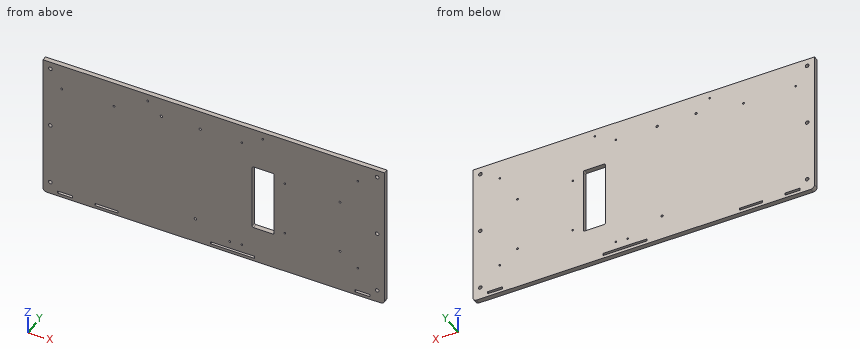
from build123d import *

# Parameters (mm, degrees)
SKETCH1_W           = 463.88
SKETCH1_H           = 192
BOSS_EXTRUDE1_DEPTH = 6.35
SKETCH5_R           = 2.5
CUT_EXTRUDE3_DEPTH  = 484.483469107
SKETCH4_R           = 1.25
SKETCH4_R_2         = 1.6
CUT_EXTRUDE2_DEPTH  = 484.483469107
SKETCH2_W           = 463.88
SKETCH2_H           = 7.175
BOSS_EXTRUDE2_DEPTH = 6.35
SKETCH3_W           = 20
SKETCH3_H           = 3.175
SKETCH3_W_2         = 31.25
SKETCH3_W_3         = 59.87
CUT_EXTRUDE1_DEPTH  = 484.483469107
FILLET1_R           = 5
SKETCH6_W           = 30
SKETCH6_H           = 92
CUT_EXTRUDE4_DEPTH  = 484.483469107
FILLET2_R           = 2


with BuildPart() as part:
    # Sketch1 → Boss-Extrude1 (new body)
    with BuildSketch(Plane(origin=(0, 0, 0), x_dir=(1, 0, 0), z_dir=(0, 1, 0))):
        with Locations((211.74, -96)):
            Rectangle(SKETCH1_W, SKETCH1_H)
    extrude(amount=-BOSS_EXTRUDE1_DEPTH)

    # Sketch5 → Cut-Extrude3 (cut, through all)
    with BuildSketch(Plane(origin=(0, 0, 0), x_dir=(1, 0, 0), z_dir=(0, 1, 0))):
        with Locations(Location((-10.2, -96, 0), (0, 0, 270))):
            Circle(SKETCH5_R)
        with Locations(Location((433.68, -96, 0), (0, 0, 270))):
            Circle(SKETCH5_R)
        with Locations(Location((-10.2, -10, 0), (0, 0, 270))):
            Circle(SKETCH5_R)
        with Locations(Location((-10.2, -182, 0), (0, 0, 270))):
            Circle(SKETCH5_R)
        with Locations(Location((433.68, -182, 0), (0, 0, 270))):
            Circle(SKETCH5_R)
        with Locations(Location((433.68, -10, 0), (0, 0, 270))):
            Circle(SKETCH5_R)
    extrude(amount=-CUT_EXTRUDE3_DEPTH, mode=Mode.SUBTRACT)

    # Sketch4 → Cut-Extrude2 (cut, through all)
    with BuildSketch(Plane(origin=(0, 0, 0), x_dir=(1, 0, 0), z_dir=(0, 1, 0))):
        with Locations(Location((407.33, -34.02, 0), (0, 0, 270))):
            Circle(SKETCH4_R)
        with Locations(Location((407.33, -166.1, 0), (0, 0, 270))):
            Circle(SKETCH4_R)
        with Locations(Location((249.85, -166.1, 0), (0, 0, 270))):
            Circle(SKETCH4_R)
        with Locations(Location((249.85, -11.16, 0), (0, 0, 270))):
            Circle(SKETCH4_R)
        with Locations(Location((186.8, -27.2, 0), (0, 0, 270))):
            Circle(SKETCH4_R_2)
        with Locations(Location((193.5, -165.7, 0), (0, 0, 270))):
            Circle(SKETCH4_R_2)
        with Locations(Location((140.6, -165.7, 0), (0, 0, 270))):
            Circle(SKETCH4_R_2)
        with Locations(Location((122.192994616, -182, 0), (0, 0, 270))):
            Circle(SKETCH4_R)
        with Locations(Location((278.192994616, -182, 0), (0, 0, 270))):
            Circle(SKETCH4_R)
        with Locations(Location((233.5, -10, 0), (0, 0, 270))):
            Circle(SKETCH4_R)
        with Locations(Location((5.25, -157, 0), (0, 0, 270))):
            Circle(SKETCH4_R)
        with Locations(Location((76.25, -157, 0), (0, 0, 270))):
            Circle(SKETCH4_R)
        with Locations(Location((308.24, -50.45, 0), (0, 0, 270))):
            Circle(SKETCH4_R)
        with Locations(Location((383.24, -50.45, 0), (0, 0, 270))):
            Circle(SKETCH4_R)
        with Locations(Location((383.24, -125.45, 0), (0, 0, 270))):
            Circle(SKETCH4_R)
        with Locations(Location((308.24, -125.45, 0), (0, 0, 270))):
            Circle(SKETCH4_R)
    extrude(amount=-CUT_EXTRUDE2_DEPTH, mode=Mode.SUBTRACT)

    # Sketch2 → Boss-Extrude2 (add)
    with BuildSketch(Plane.XZ.offset(6.35)):
        with Locations((211.74, -3.5875)):
            Rectangle(SKETCH2_W, SKETCH2_H)
    extrude(amount=-BOSS_EXTRUDE2_DEPTH)

    # Sketch3 → Cut-Extrude1 (cut, through all)
    with BuildSketch(Plane.XZ.offset(6.35)):
        with Locations((9.8, -1.5875)):
            Rectangle(SKETCH3_W, SKETCH3_H)
        with Locations((65.875, -1.5875)):
            Rectangle(SKETCH3_W_2, SKETCH3_H)
        with Locations((237.435, -1.5875)):
            Rectangle(SKETCH3_W_3, SKETCH3_H)
        with Locations((413.68, -1.5875)):
            Rectangle(SKETCH3_W, SKETCH3_H)
    extrude(amount=-CUT_EXTRUDE1_DEPTH, mode=Mode.SUBTRACT)

    # Fillet1
    fillet1_edges = [part.edges().sort_by_distance(p)[0] for p in [
        (443.68, -3.175, -7.175),
        (-20.2, -3.175, -7.175),
    ]]
    fillet(fillet1_edges, radius=FILLET1_R)

    # Sketch6 → Cut-Extrude4 (cut, through all)
    with BuildSketch(Plane(origin=(0, 0, 0), x_dir=(1, 0, 0), z_dir=(0, 1, 0))):
        with Locations((278.85, -89.18)):
            Rectangle(SKETCH6_W, SKETCH6_H)
    extrude(amount=-CUT_EXTRUDE4_DEPTH, mode=Mode.SUBTRACT)

    # Fillet2
    fillet2_edges = [part.edges().sort_by_distance(p)[0] for p in [
        (263.85, -3.175, 43.18),
        (293.85, -3.175, 43.18),
        (293.85, -3.175, 135.18),
        (263.85, -3.175, 135.18),
    ]]
    fillet(fillet2_edges, radius=FILLET2_R)


solid = part.part
The model under review builds one solid part; all positions refer to its coordinate system, in mm. Give positions to 0.01 mm unless a question says otherwise; leave off trailing zeros. Order: outer loops, then holes, each group sorted by start corner. A loop starts at its lowest first (then second) coordinate and runs counter-clockwise, first axis right, second up. Notation, with made-up numbers: M 24,32 L 83,32 A21 ccw 83,47 Z; hole C 10.25,53.25 d2. An arc over 180 degrees is marked long. Answer in a Markdown table with one row per item. Add a question column.
1. Add section A-A on z = 69.5. State the section outline as (x, y) points, plus the area to 3 significant figures.
2. To check wall thickness, follow line 1 along Z through (x, y) = (233.5, -3) (3 decimals); line 2 along Z through (x, y) = (433.68, -3.75) (3 decimals); line 3 along Z through (x, y) = (407.33, -3) (3 decimals). State the ranges of each line that lie inside material, in increasing order.
3. For pin 1 Ø2 at (x, z) = (308.24, 125.45) entering from -Y, flat-tipped, find the tip position at first contact; note if it passes through.
4. Add section B-B on y = -2.25. Count the separate pieces of the cut face and the enclosed holes in it, plus the area to 3 significant figures.
The answers:
| question | item | result |
|---|---|---|
| 1 | outline | M -20.2,-6.35 L 263.85,-6.35 L 263.85,0 L -20.2,0 Z; M 293.85,-6.35 L 443.68,-6.35 L 443.68,0 L 293.85,0 Z |
| 1 | area | 2,760 mm2 |
| 2 | line 1 | -7.175 to -3.175, 0 to 8.75, 11.25 to 192 |
| 2 | line 2 | -7.175 to 7.5, 12.5 to 93.5, 98.5 to 179.5, 184.5 to 192 |
| 2 | line 3 | -7.175 to -3.175, 0 to 32.77, 35.27 to 164.85, 167.35 to 192 |
| 3 | pin 1 | through |
| 4 | separate pieces | 1 |
| 4 | enclosed holes | 27 |
| 4 | area | 89,000 mm2 |
